```python
from build123d import *

# Parameters (mm, degrees)
SKETCH1_R           = 1.5
SKETCH1_W           = 11
SKETCH1_H           = 120
BOSS_EXTRUDE1_DEPTH = 4


with BuildPart() as part:
    # Sketch1 → Boss-Extrude1 (new body)
    with BuildSketch(Plane(origin=(0, 0, 0), x_dir=(1, 0, 0), z_dir=(0, 1, 0))):
        Polygon((-12.5, 65), (12.5, 65), (12.5, -65), (-12.5, -65), (-19.5, -65), (-19.5, -58), (-12.5, -58), (-12.5, -3.5), (-19.5, -3.5), (-19.5, 3.5), (-12.5, 3.5), (-12.5, 58), (-19.5, 58), (-19.5, 65), align=None)
        with Locations(Location((-9, 50, 0), (0, 0, 90))):
            Circle(SKETCH1_R, mode=Mode.SUBTRACT)
        with Locations(Location((-16, 61.5, 0), (0, 0, 270))):
            Circle(SKETCH1_R, mode=Mode.SUBTRACT)
        with Locations(Location((-16, 0, 0), (0, 0, 270))):
            Circle(SKETCH1_R, mode=Mode.SUBTRACT)
        with Locations(Location((-16, -61.5, 0), (0, 0, 90))):
            Circle(SKETCH1_R, mode=Mode.SUBTRACT)
        with Locations(Location((-9, -50, 0), (0, 0, 270))):
            Circle(SKETCH1_R, mode=Mode.SUBTRACT)
        with Locations(Location((-9, 30, 0), (0, 0, 90))):
            Circle(SKETCH1_R, mode=Mode.SUBTRACT)
        with Locations(Location((-9, 10, 0), (0, 0, 90))):
            Circle(SKETCH1_R, mode=Mode.SUBTRACT)
        with Locations(Location((-9, -10, 0), (0, 0, 90))):
            Circle(SKETCH1_R, mode=Mode.SUBTRACT)
        with Locations(Location((-9, -30, 0), (0, 0, 90))):
            Circle(SKETCH1_R, mode=Mode.SUBTRACT)
        Rectangle(SKETCH1_W, SKETCH1_H, mode=Mode.SUBTRACT)
    extrude(amount=BOSS_EXTRUDE1_DEPTH)


solid = part.part
```
The model under review builds one solid part; all positions refer to its coordinate system, in mm. A direction names the side the tool comes from. Give positions to 0.01 mm unless a question says otherwise; leave off trailing zeros. Write each loop counter-clockwise with the first axis right and the second up, starting at its lowest first coordinate (ties: lowest second). Pieces come first, ordered by that corner, then holes. Notation, with made-up numbers: M -3,58.25 L 47,58.25 A12 ccw 47,80.25 Z; hole C 3.25,78.25 d1. An arc over 180 degrees is marked long. Write item = value, one per line. Start each with the question number.
Q1. Machinability: for faces 4 (the face through (-16, 2, 58)), 5 (the face through (-19.5, 2, 0)), 6 (the face through (-5.5, 2, 1)), which of the approach directions +Z, -Z, +X, -X, +Y, -Y give a long, thin tool a straight path to every point of the face, cutting with its end or side? Answer none if there is none.
Q2. We need section D-D (x = -9). State the section outline as (y, z) points.
Q3. For line 1 (X direction, y = 2.25, z = 10); line 2 (X direction, y = 1.5, z = -34); line 3 (Z direction, x = -2.5, y = 3.75), list the stretches that pass through material, from the lowest coordinate up.
Q4. We need section B-B (x = 2). State the section outline as (y, z) points.
Q5. Mouldability with a two-part tool opening along X and no side actions: class faces 1 (the face through (-7, 4, -1)), 2 (the face through (12.5, 2, -1)), 3 (the face through (-9.9, 2, 48.8)) as released by +X, released by -X, zero draft, split by the parting line, or undercut.
Q6. Clearance check with flat-ended pins moving along their axes: pin 1 (10 mm diameter, centred on x = -14.5, z = -35, fed in from +Y); pin 2 (2.5 mm diameter, centred on x = -16, z = 0, fed in from +Y); pin 3 (1.2 mm diameter, centred on y = 3, z = 23, fed in from -X). State where each tip first meets the part, or that it passes through.
Q7. We need section C-C (z = -61.5). State the section outline as (x, y) points.
Q8. We need section A-A (z = 0). State the section outline as (x, y) points, plus the area to 3 significant figures.
Result set:
q1.face_4 = -X, +Y, -Y
q1.face_5 = +Z, -Z, -X, +Y, -Y
q1.face_6 = +Y, -Y
q2.outline = M 0,-65 L 4,-65 L 4,-51.5 L 0,-51.5 Z; M 0,-48.5 L 4,-48.5 L 4,-31.5 L 0,-31.5 Z; M 0,-28.5 L 4,-28.5 L 4,-11.5 L 0,-11.5 Z; M 0,-8.5 L 4,-8.5 L 4,8.5 L 0,8.5 Z; M 0,11.5 L 4,11.5 L 4,28.5 L 0,28.5 Z; M 0,31.5 L 4,31.5 L 4,48.5 L 0,48.5 Z; M 0,51.5 L 4,51.5 L 4,65 L 0,65 Z
q3.line_1 = -12.5 to -10.5, -7.5 to -5.5, 5.5 to 12.5
q3.line_2 = -12.5 to -5.5, 5.5 to 12.5
q3.line_3 = -65 to -60, 60 to 65
q4.outline = M 0,-65 L 4,-65 L 4,-60 L 0,-60 Z; M 0,60 L 4,60 L 4,65 L 0,65 Z
q5.face_1 = zero draft
q5.face_2 = released by +X
q5.face_3 = undercut
q6.pin_1 = 4
q6.pin_2 = through
q6.pin_3 = -12.5
q7.outline = M -19.5,0 L -17.5,0 L -17.5,4 L -19.5,4 Z; M -14.5,0 L 12.5,0 L 12.5,4 L -14.5,4 Z
q8.outline = M -19.5,0 L -17.5,0 L -17.5,4 L -19.5,4 Z; M -14.5,0 L -5.5,0 L -5.5,4 L -14.5,4 Z; M 5.5,0 L 12.5,0 L 12.5,4 L 5.5,4 Z
q8.area = 72.0 mm2
